The model under review builds one solid part; all positions refer to its coordinate system, in mm. Face numbers are marked on the shaded views. Give positions to 0.01 mm unless a question says otherwise; leave off trailing zeros. Order: outer loops, then holes, each group sorted by start corner. A loop starts at its lowest first (then second) coordinate and runs counter-clockwise, first axis right, second up. Notation, with made-up numbers: (33, 19.5) - (63, 19.5) arc R10 ccw to (63, 29.5) - close; hole circle Ø1 at (46, 0). An arc over 180 degrees is marked (long way). Use CSV: the item, a comma, the result in double quotes. Start each with the question number.
```python
from build123d import *

# Parameters (mm, degrees)
M3_TAPPED_HOLE1_D     = 2.5
M3_TAPPED_HOLE1_DEPTH = 4
M3_TAPPED_HOLE1_TIP   = 0.751075774


with BuildPart() as part:
    # Sketch1 → Revolve1 (revolve)
    with BuildSketch(Plane(origin=(0, 0, 0), x_dir=(0, 0, -1), z_dir=(1, 0, 0)), mode=Mode.PRIVATE) as revolve1_sk:
        Polygon((17.19, -5.15), (17.19, 5.15), (19, 5.15), (19, 6.65), (10.28, 6.65), (5.2, 6.65), (5.2, -6.65), (5.2, -11.35), (19, -11.35), (19, -5.15), align=None)
    revolve(revolve1_sk.sketch.rotate(Axis((0, 10.31552251, 0), (0, -1, 0)), 180), axis=Axis((0, 10.31552251, 0), (0, -1, 0)))

    # M3 Tapped Hole1
    with Locations(Plane(origin=(0, -11.35, 0), x_dir=(-1, 0, 0), z_dir=(0, -1, 0))):
        with Locations((0, -8), (-8, 0), (0, 8), (8, 0)):
            Hole(M3_TAPPED_HOLE1_D / 2, depth=M3_TAPPED_HOLE1_DEPTH)
            with Locations((0, 0, -(M3_TAPPED_HOLE1_DEPTH + M3_TAPPED_HOLE1_TIP / 2))):  # 118° drill point
                Cone(0, M3_TAPPED_HOLE1_D / 2, M3_TAPPED_HOLE1_TIP, mode=Mode.SUBTRACT)


solid = part.part
```
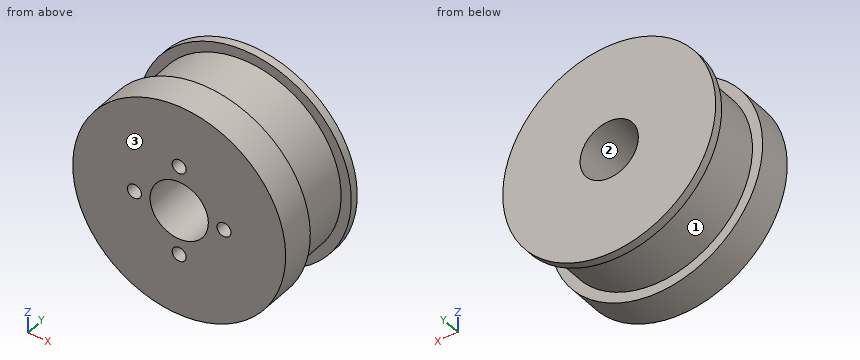
1. Consider section A-A (x = -3). Give the boundary of the cut face in (y, z), and give its area (3 significant figures).
2. Clearance check with flat-ended pins moving along their axes: pin 1 (10 mm diameter, centred on y = -8.5, z = -9, fed in from -X); pin 2 (10 mm diameter, centred on y = -5, z = -12, fed in from -X); pin 3 (1 mm diameter, centred on x = 9.5, y = -7.5, fed in from +Z); pin 4 (9.5 mm diameter, centred on x = 0, z = 0, fed in from -Y). State where each tip first meets the part, or that it passes through.
3. Consider section D-D (x = -11). Give the boundary of the cut face in (y, z), and give its area (3 significant figures).
4. Consider section B-B (z = -2). Give the boundary of the cut face in (x, y), and give its area (3 significant figures).
5. Consider section C-C (y = 4.25). Give the boundary of the cut face in (x, z).
6. To check wall thickness, follow L1, parallel to Y at x = -16.5, z = -6; L2, parallel to X at y = -5.5, z = -2; L3, parallel to Z at x = -4.5, y = -2.25. State the ranges of each line that lie inside material, in increasing order. Write a range as [from, to].
7. Mouldability with a two-part tool opening along Y and no side actions: class the marked faces 1, 2 and 3 as pulls with the +Y half, pulls with the -Y half, needs draft (parallel to the pull), parting line crosses it, or undercut.
Answers follow:
1,outline,"(-11.35, -18.76) - (-5.15, -18.76) - (-5.15, -16.93) - (5.15, -16.93) - (5.15, -18.76) - (6.65, -18.76) - (6.65, -4.25) - (-11.35, -4.25) - close; (-11.35, 4.25) - (6.65, 4.25) - (6.65, 18.76) - (5.15, 18.76) - (5.15, 16.93) - (-5.15, 16.93) - (-5.15, 18.76) - (-11.35, 18.76) - close"
1,area,"485 mm^2"
2,pin 1,"stops at x = -18.57"
2,pin 2,"stops at x = -17.66"
2,pin 3,"stops at z = 16.73"
2,pin 4,"passes through"
3,outline,"(-11.35, -15.49) - (-5.15, -15.49) - (-5.15, -13.21) - (5.15, -13.21) - (5.15, -15.49) - (6.65, -15.49) - (6.65, 15.49) - (5.15, 15.49) - (5.15, 13.21) - (-5.15, 13.21) - (-5.15, 15.49) - (-11.35, 15.49) - close"
3,area,"511 mm^2"
4,outline,"(-18.89, -11.35) - (-4.8, -11.35) - (-4.8, 6.65) - (-18.89, 6.65) - (-18.89, 5.15) - (-17.07, 5.15) - (-17.07, -5.15) - (-18.89, -5.15) - close; (4.8, -11.35) - (18.89, -11.35) - (18.89, -5.15) - (17.07, -5.15) - (17.07, 5.15) - (18.89, 5.15) - (18.89, 6.65) - (4.8, 6.65) - close"
4,area,"470 mm^2"
5,outline,"circle Ø34.38 at (0, 0); hole circle Ø10.4 at (0, 0)"
6,L1,"y = [-11.35, -5.15], [5.15, 6.65]"
6,L2,"x = [-18.89, -4.8], [4.8, 18.89]"
6,L3,"z = [-16.59, -2.61], [2.61, 16.59]"
7,face 1,"undercut"
7,face 2,"needs draft"
7,face 3,"pulls with the -Y half"
